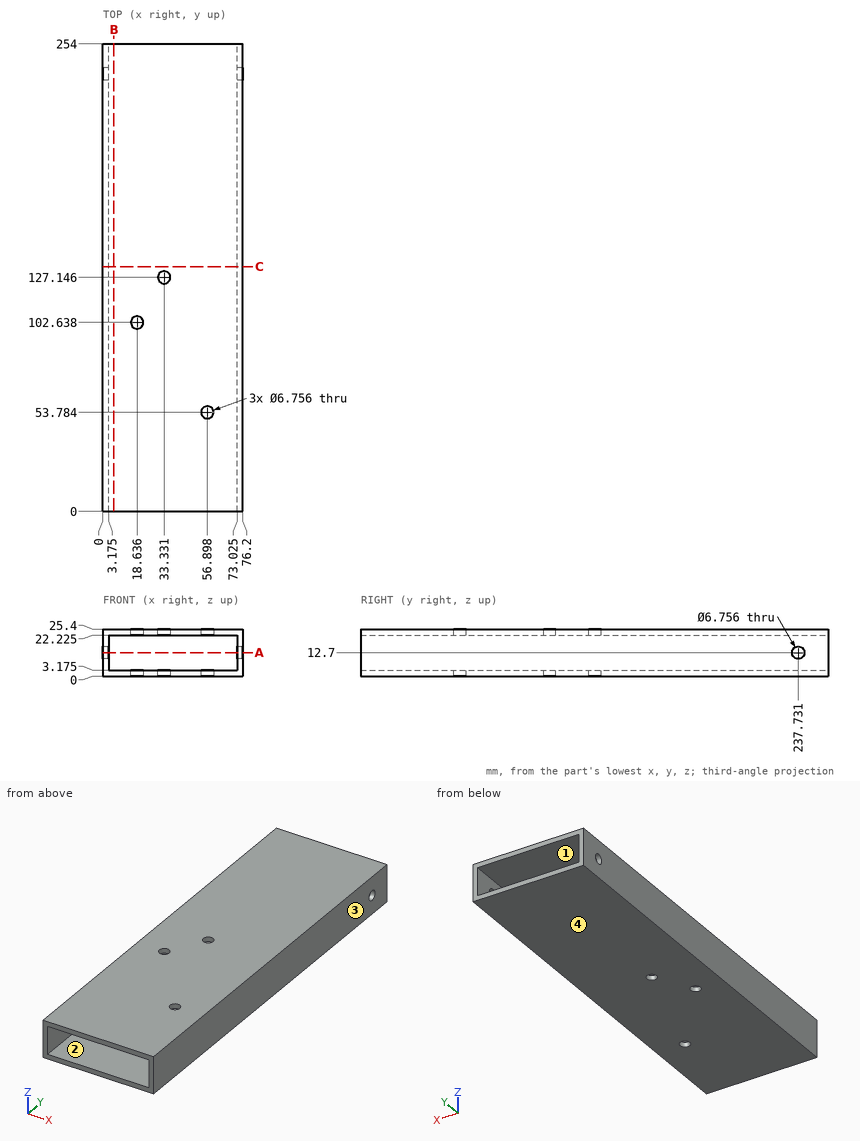
Can you work these out from the drawing? Everything is in mm from the part's minimum corner. Coordinates: 2 decimals unless noted, no trailing zeros. Loops run counter-clockwise (first coordinate to the right, second up) from the corner with the lowest first, then second, coordinate; pieces in that order, holes last. Notation, with made-up numbers: (53, -3.5) - (106, -3.5) arc R35 ccw to (106, 35.5) - close; hole circle Ø8 at (38.25, 38.5). An arc over 180 degrees is marked (long way). Use a Markdown table: item, result.
Item 1: I want a section at A-A on z = 12.7. Please give me the cut outline in (x, y) (1 decimal).
Numbers:
| item | result |
|---|---|
| outline | (0, 0) - (3.2, 0) - (3.2, 234.4) - (0, 234.4) - close; (0, 241.1) - (3.2, 241.1) - (3.2, 254) - (0, 254) - close; (73, 0) - (76.2, 0) - (76.2, 234.4) - (73, 234.4) - close; (73, 241.1) - (76.2, 241.1) - (76.2, 254) - (73, 254) - close |
Item 2: If I drill on probe 1 along Z at (x, y) = (62.5, 32.5) (1 decimal); probe 2 along X at (y, z) = (149, 15.5) (1 decimal); probe 3 along Y at (x, z) = (74.7, 12.7), over which ranges is the centre line in solid material (lowest first)? Write a range as from..to.
Numbers:
| item | result |
|---|---|
| probe 1 | z = 0..3.2, 22.2..25.4 |
| probe 2 | x = 0..3.2, 73..76.2 |
| probe 3 | y = 0..234.35, 241.11..254 |
Item 3: I want a section at C-C on y = 133. Please give me the cut outline in (x, z) (1 decimal).
Numbers:
| item | result |
|---|---|
| outline | (0, 0) - (76.2, 0) - (76.2, 25.4) - (0, 25.4) - close; hole (3.2, 3.2) - (73, 3.2) - (73, 22.2) - (3.2, 22.2) - close |
Item 4: I want a section at B-B on x = 6. Please give me the cut outline in (y, z) (1 decimal), and give its area (3 significant figures).
Numbers:
| item | result |
|---|---|
| outline | (0, 0) - (254, 0) - (254, 3.2) - (0, 3.2) - close; (0, 22.2) - (254, 22.2) - (254, 25.4) - (0, 25.4) - close |
| area | 1,610 mm2 |
Item 5: We'd pull the mould along X, two halves only. Please class the marked faces 1, 2, 3 and 4: released by +X, released by -X, zero draft, split by the parting line, or undercut.
Numbers:
| item | result |
|---|---|
| face 1 | undercut |
| face 2 | undercut |
| face 3 | released by +X |
| face 4 | zero draft |
Item 6: Will these pins go through, and if not, where does the flat tip stop? pin 1 (21 mm diameter, centred on x = 40, y = 149, fed in from -Z); pin 2 (5.5 mm diameter, centred on x = 18.64, y = 102.64, fed in from +Z).
Numbers:
| item | result |
|---|---|
| pin 1 | stops at z = 0 |
| pin 2 | passes through |
